from build123d import *

# Parameters (mm, degrees)
BOSS_EXTRUDE1_DEPTH              = 50.8
F_6_32_TAPPED_HOLE1_AT_2_COUNT   = 2
F_6_32_TAPPED_HOLE1_AT_2_PITCH   = 40.005
F_6_32_TAPPED_HOLE1_AT_3_COUNT   = 2
F_6_32_TAPPED_HOLE1_AT_3_PITCH   = 179.52019402
F_6_32_TAPPED_HOLE1_AT_4_COUNT   = 2
F_6_32_TAPPED_HOLE1_AT_4_PITCH   = 175.006
BOSS_EXTRUDE2_DEPTH              = 61.976
CUT_EXTRUDE2_DEPTH               = 20.05
F_8_32_TAPPED_HOLE1_AT_2_COUNT   = 2
F_8_32_TAPPED_HOLE1_AT_2_PITCH   = 62.357
F_8_32_TAPPED_HOLE1_AT_3_COUNT   = 2
F_8_32_TAPPED_HOLE1_AT_3_PITCH   = 185.065844998
F_8_32_TAPPED_HOLE1_AT_4_COUNT   = 2
F_8_32_TAPPED_HOLE1_AT_4_PITCH   = 174.244
F_8_32_TAPPED_HOLE1_AT_5_COUNT   = 2
F_8_32_TAPPED_HOLE1_AT_5_PITCH   = 87.122
SKETCH13_W                       = 162.052
SKETCH13_H                       = 63.881
BOSS_EXTRUDE4_DEPTH              = 4.318
F_8_32_TAPPED_HOLE2_AT_2_COUNT   = 2
F_8_32_TAPPED_HOLE2_AT_2_PITCH   = 41.171214069
F_8_32_TAPPED_HOLE2_AT_3_COUNT   = 2
F_8_32_TAPPED_HOLE2_AT_3_PITCH   = 87.455597175
F_8_32_TAPPED_HOLE2_AT_4_COUNT   = 2
F_8_32_TAPPED_HOLE2_AT_4_PITCH   = 81.8388
F_8_32_TAPPED_HOLE2_AT_5_COUNT   = 2
F_8_32_TAPPED_HOLE2_AT_5_PITCH   = 57.868770444
F_8_32_TAPPED_HOLE2_AT_6_COUNT   = 2
F_8_32_TAPPED_HOLE2_AT_6_PITCH   = 41.171214069
CUT_EXTRUDE3_DEPTH               = 3.54
F_1_4_20_TAPPED_HOLE1_AT_2_COUNT = 2
F_1_4_20_TAPPED_HOLE1_AT_2_PITCH = 50.8


with BuildPart() as part:
    # Sketch1 → Boss-Extrude1 (new body)
    with BuildSketch(Plane.XY):
        Polygon((-92.71, 2.54), (92.71, 2.54), (92.71, 0), (113.03, 0), (113.03, 19.05), (92.71, 19.05), (92.71, 74.93), (-92.71, 74.93), (-92.71, 19.05), (-113.03, 19.05), (-113.03, 0), (-92.71, 0), align=None)
    extrude(amount=-BOSS_EXTRUDE1_DEPTH)

    # Sketch3 → #6-32 Tapped Hole1 (revolve, cut)
    with BuildSketch(Plane(origin=(-87.503, 74.93, -45.4025), x_dir=(0, 0, 1), z_dir=(1, 0, 0))):
        Polygon((0, 0), (0, 14.42709403), (1.35255, 13.6144), (1.35255, 9.652), (1.7526, 9.652), (1.7526, 0.635), (2.3876, 0), align=None)
    f_6_32_tapped_hole1 = revolve(axis=Axis((-87.503, 81.28, -45.4025), (0, -1, 0)), mode=Mode.SUBTRACT)

    # #6-32 Tapped Hole1 at 2: #6-32 Tapped Hole1 ×2
    with Locations(*[(0, 0, i * F_6_32_TAPPED_HOLE1_AT_2_PITCH) for i in range(1, F_6_32_TAPPED_HOLE1_AT_2_COUNT)]):
        add(f_6_32_tapped_hole1, mode=Mode.SUBTRACT)

    # #6-32 Tapped Hole1 at 3: #6-32 Tapped Hole1 ×2
    with Locations(*[Vector(0.974854116, 0, 0.22284401) * (i * F_6_32_TAPPED_HOLE1_AT_3_PITCH) for i in range(1, F_6_32_TAPPED_HOLE1_AT_3_COUNT)]):
        add(f_6_32_tapped_hole1, mode=Mode.SUBTRACT)

    # #6-32 Tapped Hole1 at 4: #6-32 Tapped Hole1 ×2
    with Locations(*[(i * F_6_32_TAPPED_HOLE1_AT_4_PITCH, 0, 0) for i in range(1, F_6_32_TAPPED_HOLE1_AT_4_COUNT)]):
        add(f_6_32_tapped_hole1, mode=Mode.SUBTRACT)

    # Sketch5 → Boss-Extrude2 (add)
    with BuildSketch(Plane.XY):
        Polygon((92.71, 74.93), (-92.71, 74.93), (-92.71, 19.05), (-113.03, 19.05), (-113.03, 0), (113.03, 0), (113.03, 19.05), (92.71, 19.05), align=None)
    extrude(amount=BOSS_EXTRUDE2_DEPTH)

    # Sketch16 → Cut-Extrude2 (cut, through all)
    with BuildSketch(Plane(origin=(0, 19.05, 0), x_dir=(1, 0, 0), z_dir=(0, 1, 0))):
        with BuildLine():
            Line((-104.9782, 38.1), (-104.9782, -12.7))
            ThreePointArc((-104.9782, -12.7), (-101.6, -16.0782), (-98.2218, -12.7))
            Line((-98.2218, -12.7), (-98.2218, 38.1))
            ThreePointArc((-98.2218, 38.1), (-101.6, 41.4782), (-104.9782, 38.1))
        make_face()
        with BuildLine():
            Line((104.9782, 38.1), (104.9782, -12.7))
            ThreePointArc((104.9782, -12.7), (101.6, -16.0782), (98.2218, -12.7))
            Line((98.2218, -12.7), (98.2218, 38.1))
            ThreePointArc((98.2218, 38.1), (101.6, 41.4782), (104.9782, 38.1))
        make_face()
    extrude(amount=-CUT_EXTRUDE2_DEPTH, mode=Mode.SUBTRACT)

    # Sketch11 → #8-32 Tapped Hole1 (revolve, cut)
    with BuildSketch(Plane(origin=(-87.122, 69.977, 61.976), x_dir=(0, -1, 0), z_dir=(1, 0, 0))):
        Polygon((0, 0), (0, 17.700206461), (1.7272, 16.6624), (1.7272, 12.7), (2.0828, 12.7), (2.0828, 0.635), (2.7178, 0), align=None)
    f_8_32_tapped_hole1 = revolve(axis=Axis((-87.122, 69.977, 68.326), (0, 0, -1)), mode=Mode.SUBTRACT)

    # #8-32 Tapped Hole1 at 2: #8-32 Tapped Hole1 ×2
    with Locations(*[(0, -i * F_8_32_TAPPED_HOLE1_AT_2_PITCH, 0) for i in range(1, F_8_32_TAPPED_HOLE1_AT_2_COUNT)]):
        add(f_8_32_tapped_hole1, mode=Mode.SUBTRACT)

    # #8-32 Tapped Hole1 at 3: #8-32 Tapped Hole1 ×2
    with Locations(*[Vector(0.941524353, -0.33694494, 0) * (i * F_8_32_TAPPED_HOLE1_AT_3_PITCH) for i in range(1, F_8_32_TAPPED_HOLE1_AT_3_COUNT)]):
        add(f_8_32_tapped_hole1, mode=Mode.SUBTRACT)

    # #8-32 Tapped Hole1 at 4: #8-32 Tapped Hole1 ×2
    with Locations(*[(i * F_8_32_TAPPED_HOLE1_AT_4_PITCH, 0, 0) for i in range(1, F_8_32_TAPPED_HOLE1_AT_4_COUNT)]):
        add(f_8_32_tapped_hole1, mode=Mode.SUBTRACT)

    # #8-32 Tapped Hole1 at 5: #8-32 Tapped Hole1 ×2
    with Locations(*[(i * F_8_32_TAPPED_HOLE1_AT_5_PITCH, 0, 0) for i in range(1, F_8_32_TAPPED_HOLE1_AT_5_COUNT)]):
        add(f_8_32_tapped_hole1, mode=Mode.SUBTRACT)

    # Sketch13 → Boss-Extrude4 (add)
    with BuildSketch(Plane.XY.offset(61.976)):
        with Locations((0, 31.9405)):
            Rectangle(SKETCH13_W, SKETCH13_H)
    extrude(amount=BOSS_EXTRUDE4_DEPTH)

    # Sketch7 → #8-32 Tapped Hole2 (revolve, cut)
    with BuildSketch(Plane(origin=(-40.9194, 52.4002, 66.294), x_dir=(0, -1, 0), z_dir=(1, 0, 0))):
        Polygon((0, 0), (0, 17.700206461), (1.7272, 16.6624), (1.7272, 12.7), (2.0828, 12.7), (2.0828, 0.635), (2.7178, 0), align=None)
    f_8_32_tapped_hole2 = revolve(axis=Axis((-40.9194, 52.4002, 72.644), (0, 0, -1)), mode=Mode.SUBTRACT)

    # #8-32 Tapped Hole2 at 2: #8-32 Tapped Hole2 ×2
    with Locations(*[Vector(0.110431526, -0.993883735, 0) * (i * F_8_32_TAPPED_HOLE2_AT_2_PITCH) for i in range(1, F_8_32_TAPPED_HOLE2_AT_2_COUNT)]):
        add(f_8_32_tapped_hole2, mode=Mode.SUBTRACT)

    # #8-32 Tapped Hole2 at 3: #8-32 Tapped Hole2 ×2
    with Locations(*[Vector(0.883787916, -0.46788772, 0) * (i * F_8_32_TAPPED_HOLE2_AT_3_PITCH) for i in range(1, F_8_32_TAPPED_HOLE2_AT_3_COUNT)]):
        add(f_8_32_tapped_hole2, mode=Mode.SUBTRACT)

    # #8-32 Tapped Hole2 at 4: #8-32 Tapped Hole2 ×2
    with Locations(*[(i * F_8_32_TAPPED_HOLE2_AT_4_PITCH, 0, 0) for i in range(1, F_8_32_TAPPED_HOLE2_AT_4_COUNT)]):
        add(f_8_32_tapped_hole2, mode=Mode.SUBTRACT)

    # #8-32 Tapped Hole2 at 5: #8-32 Tapped Hole2 ×2
    with Locations(*[Vector(0.707106781, -0.707106781, 0) * (i * F_8_32_TAPPED_HOLE2_AT_5_PITCH) for i in range(1, F_8_32_TAPPED_HOLE2_AT_5_COUNT)]):
        add(f_8_32_tapped_hole2, mode=Mode.SUBTRACT)

    # #8-32 Tapped Hole2 at 6: #8-32 Tapped Hole2 ×2
    with Locations(*[Vector(0.993883735, -0.110431526, 0) * (i * F_8_32_TAPPED_HOLE2_AT_6_PITCH) for i in range(1, F_8_32_TAPPED_HOLE2_AT_6_COUNT)]):
        add(f_8_32_tapped_hole2, mode=Mode.SUBTRACT)

    # Sketch17 → Cut-Extrude3 (cut, through all)
    with BuildSketch(Plane.XZ.offset(-2.54)):
        with BuildLine():
            Line((-92.71, 0), (92.71, 0))
            Line((92.71, 0), (92.71, 49.403))
            ThreePointArc((92.71, 49.403), (89.920192091, 56.138192091), (83.185, 58.928))
            Line((83.185, 58.928), (-83.185, 58.928))
            ThreePointArc((-83.185, 58.928), (-89.920192091, 56.138192091), (-92.71, 49.403))
            Line((-92.71, 49.403), (-92.71, 0))
        make_face()
    extrude(amount=CUT_EXTRUDE3_DEPTH, mode=Mode.SUBTRACT)

    # Sketch18 → 1/4-20 Tapped Hole1 (revolve, cut)
    with BuildSketch(Plane(origin=(25.4, 38.1, -50.8), x_dir=(0, 1, 0), z_dir=(1, 0, 0))):
        Polygon((0, 0), (0, 20.583816902), (2.5527, 19.05), (2.5527, 12.7), (3.175, 12.7), (3.175, 0.762), (3.937, 0), align=None)
    f_1_4_20_tapped_hole1 = revolve(axis=Axis((25.4, 38.1, -57.15), (0, 0, 1)), mode=Mode.SUBTRACT)

    # 1/4-20 Tapped Hole1 at 2: 1/4-20 Tapped Hole1 ×2
    with Locations(*[(-i * F_1_4_20_TAPPED_HOLE1_AT_2_PITCH, 0, 0) for i in range(1, F_1_4_20_TAPPED_HOLE1_AT_2_COUNT)]):
        add(f_1_4_20_tapped_hole1, mode=Mode.SUBTRACT)


solid = part.part
Verification items for the finished model (mm, model axes). A direction names the side the tool comes from. Round coordinates to 2 decimals unless told otherwise and drop trailing zeros. Loops run counter-clockwise (first coordinate to the right, second up) from the corner with the lowest first, then second, coordinate; pieces in that order, holes last. Notation, with made-up numbers: (24, 66.5) - (68, 66.5) arc R15 cw to (68, 95.5) - close; hole circle Ø11 at (86, -15). An arc over 180 degrees is marked (long way). Use one line per item in the form item = value.
1. Section check A-A on x = -101.6. Record the cut outline in (y, z), and give its area (3 significant figures).
A:
outline = (0, -50.8) - (19.05, -50.8) - (19.05, -41.48) - (0, -41.48) - close; (0, 16.08) - (19.05, 16.08) - (19.05, 61.98) - (0, 61.98) - close
area = 1,050 mm²
2. Section check B-B on z = -27. Record the cut outline in (x, y), and give its area (3 significant figures).
A:
outline = (-113.03, 0) - (-104.98, 0) - (-104.98, 19.05) - (-113.03, 19.05) - close; (-98.22, 0) - (-92.71, 0) - (-92.71, 2.54) - (92.71, 2.54) - (92.71, 0) - (98.22, 0) - (98.22, 19.05) - (92.71, 19.05) - (92.71, 74.93) - (-92.71, 74.93) - (-92.71, 19.05) - (-98.22, 19.05) - close; (104.98, 0) - (113.03, 0) - (113.03, 19.05) - (104.98, 19.05) - close
area = 13,900 mm²
3. Section check D-D on x = 75.5. Record the cut outline in (y, z).
A:
outline = (0, 58.93) - (2.54, 58.93) - (2.54, -50.8) - (74.93, -50.8) - (74.93, 61.98) - (63.88, 61.98) - (63.88, 66.29) - (0, 66.29) - close
4. Access from +Z, -Z, +X, -X, +Y, -Y to the whole of each face (thin tool, end or side, straight path). Record for faces 5 (the flat face through (-1, 63.881, 64)), 6 (the cylindrical face through (-89.85, 1.29, 56.21)), 7 (the flat face through (81.026, 31, 64)), 8 (the flat face through (-81.026, 31, 64)), 9 (the cylindrical face through (27.665, 39.278, -34.969)).
A:
face_5 = +Z, +X, -X, +Y
face_6 = -Z, -Y
face_7 = +Z, +X, +Y, -Y
face_8 = +Z, -X, +Y, -Y
face_9 = -Z
5. Scan lines: probe 1 along X at (y, z) = (53.5, 60.5); probe 2 along X at (y, z) = (38.1, -43.5) (3 decimals); probe 3 along Y at (x, z) = (0, 47). Record each from-to range of solid material in increasing order.
A:
probe_1 = -92.71 to -42.69, -39.15 to 39.15, 42.69 to 92.71
probe_2 = -92.71 to -28.575, -22.225 to 22.225, 28.575 to 92.71
probe_3 = 2.54 to 68.25, 71.7 to 74.93
6. Section check C-C on y = 30. Record the cut outline in (x, z).
A:
outline = (-92.71, -50.8) - (92.71, -50.8) - (92.71, 61.98) - (81.03, 61.98) - (81.03, 66.29) - (-81.03, 66.29) - (-81.03, 61.98) - (-92.71, 61.98) - close
7. Draft check along Z on faces 1 (the flat face through (-89, 70, 49.276)), 2 (the cylindrical face through (-101.526, 9.658, -41.477)), 3 (the cylindrical face through (23.254, 35.76, -44.153)), 4 (the cylindrical face through (101.674, 9.658, 16.077)). Enter one of: pulls with the +Z half, pulls with the -Z half, needs draft (parallel to the pull), parting line crosses it, or undercut.
A:
face_1 = pulls with the +Z half
face_2 = undercut
face_3 = needs draft
face_4 = undercut
8. Gauge pin test, flat ends, axial feed: pin 1 Ø4 at (y, z) = (46.5, 12) entering from -X; pin 2 Ø2 at (x, y) = (87.122, 7.62) entering from +Z; pin 3 Ø1.3 at (x, y) = (-3.5, 1.5) entering from -Z. Record the tip position at first contact, or that the pin passes through.
A:
pin_1 = -92.71
pin_2 = 44.88
pin_3 = 58.93
